Design review of the part built by this model. Coordinates are the model's own, in mm. Give positions to 0.01 mm unless a question says otherwise; leave off trailing zeros. Order: outer loops, then holes, each group sorted by start corner. A loop starts at its lowest first (then second) coordinate and runs counter-clockwise, first axis right, second up. Notation, with made-up numbers: (18.5, 85) -> (26.5, 85) arc R20 cw to (26.5, 96) -> close; hole circle Ø8 at (52, 43). An arc over 180 degrees is marked (long way). Use a Markdown table: item, result. Add a question column.
```python
from build123d import *

# Parameters (mm, degrees)
BOSS_EXTRUDE1_DEPTH         = 3.175
F_1_4_0_25_DIAMETER_HOLE1_D = 6.35
F_1_4_CLEARANCE_HOLE1_D     = 6.7564


with BuildPart() as part:
    # Sketch1 → Boss-Extrude1 (new body)
    with BuildSketch(Plane(origin=(0, 0, 0), x_dir=(1, 0, 0), z_dir=(0, 1, 0))):
        Polygon((-330.2, 0), (-154.051, 321.128911223), (154.051, 321.128911223), (330.2, 0), align=None)
    extrude(amount=BOSS_EXTRUDE1_DEPTH)

    # 1/4 (0.25) Diameter Hole1 (through all)
    with Locations(Plane(origin=(0, 3.175, 0), x_dir=(1, 0, 0), z_dir=(0, 1, 0))):
        with Locations((-279.364444826, 66.268686649), (-178.463561331, 250.216315407), (-101.6, 308.428911223), (279.364444826, 66.268686649), (178.463561331, 250.216315407), (101.6, 308.428911223)):
            Hole(F_1_4_0_25_DIAMETER_HOLE1_D / 2)

    # 1/4 Clearance Hole1 (through all)
    with Locations(Plane(origin=(0, 3.175, 0), x_dir=(1, 0, 0), z_dir=(0, 1, 0))):
        with Locations((-123.952, 250.216315407), (-244.348, 50.8), (244.348, 50.8), (123.952, 250.216315407)):
            Hole(F_1_4_CLEARANCE_HOLE1_D / 2)


solid = part.part
```
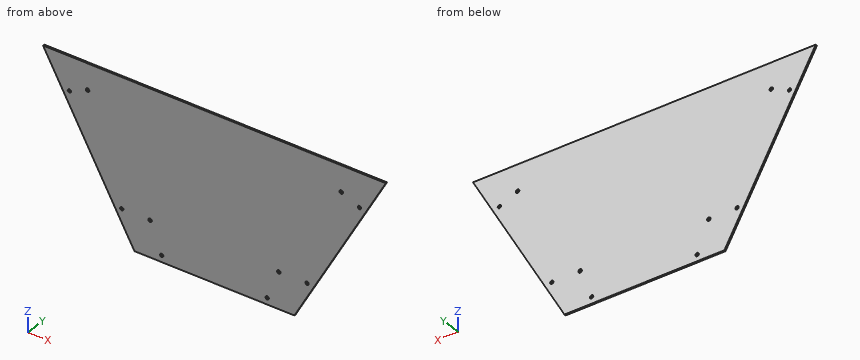
1) Insertion check: pin 1 (5 mm diameter, centred on x = 178.46, z = -250.22, fed in from -Y); pin 2 (1.5 mm diameter, centred on y = 2.5, z = -284, fed in from +X). Each pin has a flat end and moves straight along its axis. Give the tip position at first contact, or say it passes through.
2) For L1, parallel to Z at x = -101.6, y = 1; L2, parallel to Z at x = -264, y = 1.5; L3, parallel to Z at x = -190.5, y = 1.05, list the stretches that pass through material, from the lowest coordinate up. Write a range as [from, to].
3) Add section B-B (x = -289). Give the boundary of the cut face in (y, z) (3 decimals).
4) Add section A-A (y = 1.15). Give the number of separate pieces and of enclosed holes in the cut face, then the cut area to 3 significant figures.
Worked answers:
| question | item | result |
|---|---|---|
| 1 | pin 1 | through |
| 1 | pin 2 | x = 174.83 |
| 2 | L1 | [-321.13, -311.6], [-305.25, 0] |
| 2 | L2 | [-120.69, 0] |
| 2 | L3 | [-254.68, 0] |
| 3 | outline | (0, -75.11) -> (3.175, -75.11) -> (3.175, 0) -> (0, 0) -> close |
| 4 | separate pieces | 1 |
| 4 | enclosed holes | 10 |
| 4 | area | 155,000 mm^2 |
